```python
from build123d import *

# Parameters (mm, degrees)
F0_W     = 223.13392
F0_H     = 14.8336
F1_DEPTH = 9.525
F2_R     = 2.54
F3_DEPTH = 9.526
F4_W     = 10.795
F4_H     = 14.8336
F5_DEPTH = 6.35
F7_DEPTH = 12.7
F8_R     = 5.08


with BuildPart() as f1:
    # F0 (on Top) → F1 (new body)
    with BuildSketch(Plane.XY):
        with Locations((0, 7.62)):
            Rectangle(F0_W, F0_H)
    extrude(amount=F1_DEPTH)

    # F2 (on face) → F3 (cut, through all)
    with BuildSketch(Plane.XY.offset(9.525)):
        with Locations((-81.28, 5.08)):
            Circle(F2_R)
        with Locations((81.28, 5.08)):
            Circle(F2_R)
    extrude(amount=-F3_DEPTH, mode=Mode.SUBTRACT)

    # F4 (on face) → F5 (join)
    with BuildSketch(Plane(origin=(0, 0, 0), x_dir=(1, 0, 0), z_dir=(0, 0, -1))):
        with Locations((-106.16946, -7.62)):
            Rectangle(F4_W, F4_H)
        with Locations((106.16946, -7.62)):
            Rectangle(F4_W, F4_H)
    extrude(amount=F5_DEPTH)

    # F6 (on face) → F7 (join)
    with BuildSketch(Plane.XZ.offset(-0.2032)):
        Polygon((100.77196, -6.35), (111.56696, -6.35), (111.56696, 9.525), (-111.56696, 9.525), (-111.56696, -6.35), (-100.77196, -6.35), (-100.77196, 0), (100.77196, 0), align=None)
    extrude(amount=F7_DEPTH)

    # F8
    f8_edges = [f1.edges().sort_by_distance(p)[0] for p in [
        (111.56696, -12.4968, 1.5875),
        (111.56696, 15.0368, 1.5875),
        (-111.56696, -12.4968, 1.5875),
        (-111.56696, 15.0368, 1.5875),
    ]]
    fillet(f8_edges, radius=F8_R)


solid = f1.part
```
Geometry: final body of the model. Coordinates: model frame, mm. A direction names the side the tool comes from. Round coordinates to 2 decimals unless told otherwise and drop trailing zeros. Order: outer loops, then holes, each group sorted by start corner. A loop starts at its lowest first (then second) coordinate and runs counter-clockwise, first axis right, second up. Notation, with made-up numbers: (79, -20) -> (115, -20) arc R8 cw to (115, -9) -> close; hole circle Ø4 at (-23, -5.5). An arc over 180 degrees is marked (long way). Use CSV: the item, a comma, the result in double quotes. Start each with the question number.
1) Section A-A (y = 5.08). Return the cut outline in (x, z) (3 decimals).
2) First-contact query: pin 1 Ø3 at (x, y) = (81.28, 5.08) entering from -Z; pin 2 Ø6 at (x, y) = (-81.28, 5.08) entering from -Z; pin 3 Ø4 at (y, z) = (-9.5, 5.5) entering from -X. Flat tips, straight axial feed; report the tip coordinate or a pass-through.
3) Material intervals for line 1 along Y through (x, z) = (81.28, 3); line 2 along X through (y, z) = (4.75, -5); line 3 along Z through (x, y) = (49, 0.5) (3 decimals), sorted ascending. Write a range as from..to.
4) Section C-C (x = 81.28). Return the cut outline in (y, z) (3 decimals), and give its area (3 significant figures).
5) Set-up query: faces 1 (the face through (100.772, 1, -3)), 2 (the face through (-106, 1, -6.35)). Return all of +Z, -Z, +X, -X, +Y, -Y with unobstructed straight access to the full face (end or side cutting, diameter ignored); none if empty.
6) Draft query along X for faces 3 (the face through (-100.772, 1, -3)), 4 (the face through (106, 1, -6.35)), 5 (the face through (-111.567, 1, 2)). Return one class per face: +X half, -X half, draft (parallel to the pull), parting line (faces both ways), or undercut.
7) Section B-B (z = -4.5). Return the cut outline in (x, y).
Returned:
1,outline,"(-111.567, -6.35) -> (-100.772, -6.35) -> (-100.772, 0) -> (-83.82, 0) -> (-83.82, 9.525) -> (-111.567, 9.525) -> close; (-78.74, 0) -> (78.74, 0) -> (78.74, 9.525) -> (-78.74, 9.525) -> close; (83.82, 0) -> (100.772, 0) -> (100.772, -6.35) -> (111.567, -6.35) -> (111.567, 9.525) -> (83.82, 9.525) -> close"
2,pin 1,"passes through"
2,pin 2,"stops at z = 0"
2,pin 3,"stops at x = -111.57"
3,line 1,"y = -12.5..2.54, 7.62..15.04"
3,line 2,"x = -111.57..-100.77, 100.77..111.57"
3,line 3,"z = 0..9.525"
4,outline,"(-12.497, 0) -> (2.54, 0) -> (2.54, 9.525) -> (-12.497, 9.525) -> close; (7.62, 0) -> (15.037, 0) -> (15.037, 9.525) -> (7.62, 9.525) -> close"
4,area,"214 mm²"
5,face 1,"-Z, +Y, -Y"
5,face 2,"-Z, +X, -X, +Y, -Y"
6,face 3,"undercut"
6,face 4,"draft"
6,face 5,"-X half"
7,outline,"(-111.57, -7.42) arc R5.08 ccw to (-106.49, -12.5) -> (-100.77, -12.5) -> (-100.77, 15.04) -> (-106.49, 15.04) arc R5.08 ccw to (-111.57, 9.96) -> close; (100.77, -12.5) -> (106.49, -12.5) arc R5.08 ccw to (111.57, -7.42) -> (111.57, 9.96) arc R5.08 ccw to (106.49, 15.04) -> (100.77, 15.04) -> close"
